from build123d import *

# Parameters (mm, degrees)
SKETCH1_W           = 35.999968648
SKETCH1_H           = 39.60056603
BOSS_EXTRUDE1_DEPTH = 33.93
SKETCH2_W           = 28.93
SKETCH2_H           = 5
SKETCH2_H_2         = 4
CUT_EXTRUDE1_DEPTH  = 64.367558518
SKETCH3_W           = 16
SKETCH3_H           = 5
SKETCH3_H_2         = 4
CUT_EXTRUDE2_DEPTH  = 64.367558518
CUT_EXTRUDE3_DEPTH  = 61.369212453
SKETCH5_W           = 30.4
SKETCH5_H           = 7.2
CUT_EXTRUDE4_DEPTH  = 30.93
CUT_EXTRUDE5_DEPTH  = 62.813165851
BOSS_EXTRUDE2_REACH = 65.368
BOSS_EXTRUDE3_DEPTH = 5
BOSS_EXTRUDE4_REACH = 56.06
BOSS_EXTRUDE5_DEPTH = 5
BOSS_EXTRUDE6_DEPTH = 3
SKETCH12_W          = 35.999968648
SKETCH12_H          = 45.60056603
CUT_EXTRUDE6_DEPTH  = 2
SKETCH13_W          = 30.4
SKETCH13_H          = 39.6
SKETCH13_W_2        = 29.9
SKETCH13_H_2        = 39.1
CUT_EXTRUDE7_DEPTH  = 2


with BuildPart() as part:
    # Sketch1 → Boss-Extrude1 (new body)
    with BuildSketch(Plane.XY):
        with Locations((17.999984324, 19.800283015)):
            Rectangle(SKETCH1_W, SKETCH1_H)
    extrude(amount=-BOSS_EXTRUDE1_DEPTH)

    # Sketch2 → Cut-Extrude1 (cut, through all)
    with BuildSketch(Plane(origin=(35.999968648, 0, 0), x_dir=(0, 0, -1), z_dir=(1, 0, 0))):
        with Locations((19.465, 37.10056603)):
            Rectangle(SKETCH2_W, SKETCH2_H)
        with Locations((19.465, 19.800283015)):
            Rectangle(SKETCH2_W, SKETCH2_H_2)
        with Locations((19.465, 2.5)):
            Rectangle(SKETCH2_W, SKETCH2_H)
    extrude(amount=-CUT_EXTRUDE1_DEPTH, mode=Mode.SUBTRACT)

    # Sketch3 → Cut-Extrude2 (cut, through all)
    with BuildSketch(Plane.XY):
        with Locations((17.999984324, 37.10056603)):
            Rectangle(SKETCH3_W, SKETCH3_H)
        with Locations((17.999984324, 19.800283015)):
            Rectangle(SKETCH3_W, SKETCH3_H_2)
        with Locations((17.999984324, 2.5)):
            Rectangle(SKETCH3_W, SKETCH3_H)
    extrude(amount=-CUT_EXTRUDE2_DEPTH, mode=Mode.SUBTRACT)

    # Sketch4 → Cut-Extrude3 (cut, through all)
    with BuildSketch(Plane(origin=(0, 34.60056603, 0), x_dir=(1, 0, 0), z_dir=(0, 1, 0))):
        Polygon((9.999984324, 0), (17.999984324, 5), (25.999984324, 0), align=None)
    extrude(amount=-CUT_EXTRUDE3_DEPTH, mode=Mode.SUBTRACT)

    # Sketch5 → Cut-Extrude4 (cut)
    with BuildSketch(Plane.XY):
        with Locations((17.999984324, 11.4)):
            Rectangle(SKETCH5_W, SKETCH5_H)
        with Locations((17.999984324, 28.20056603)):
            Rectangle(SKETCH5_W, SKETCH5_H)
    extrude(amount=-CUT_EXTRUDE4_DEPTH, mode=Mode.SUBTRACT)

    # Sketch6 → Cut-Extrude5 (cut, through all)
    with BuildSketch(Plane.XY.offset(-30.93)):
        with BuildLine():
            Line((15.109984324, 29.66056603), (20.889984324, 29.66056603))
            ThreePointArc((20.889984324, 29.66056603), (22.469984324, 28.08056603), (20.889984324, 26.50056603))
            Line((20.889984324, 26.50056603), (15.109984324, 26.50056603))
            ThreePointArc((15.109984324, 26.50056603), (13.529984324, 28.08056603), (15.109984324, 29.66056603))
        make_face()
        with BuildLine():
            Line((15.109984324, 12.86), (20.889984324, 12.86))
            ThreePointArc((20.889984324, 12.86), (22.469984324, 11.28), (20.889984324, 9.7))
            Line((20.889984324, 9.7), (15.109984324, 9.7))
            ThreePointArc((15.109984324, 9.7), (13.529984324, 11.28), (15.109984324, 12.86))
        make_face()
    extrude(amount=-CUT_EXTRUDE5_DEPTH, mode=Mode.SUBTRACT)

    # Sketch7 → Boss-Extrude2 (add, up to next)
    with BuildSketch(Plane.XY, mode=Mode.PRIVATE) as boss_extrude2_sk1:
        Polygon((2.799984324, 28.422935376), (2.799984324, 27.45056603), (3.299984324, 27.45056603), (3.299984324, 27.896781183), align=None)
    boss_extrude2_tool1 = extrude(boss_extrude2_sk1.sketch, amount=-BOSS_EXTRUDE2_REACH, mode=Mode.PRIVATE) - part.part
    # Sketch7 → Boss-Extrude2 (add, up to next)
    with BuildSketch(Plane.XY, mode=Mode.PRIVATE) as boss_extrude2_sk2:
        Polygon((2.799984324, 11.622369346), (2.799984324, 10.65), (3.299984324, 10.65), (3.299984324, 11.096215154), align=None)
    boss_extrude2_tool2 = extrude(boss_extrude2_sk2.sketch, amount=-BOSS_EXTRUDE2_REACH, mode=Mode.PRIVATE) - part.part
    boss_extrude2_1 = boss_extrude2_tool1.solids().sort_by_distance((3.019076, 27.821475, 0))[0]
    add(boss_extrude2_1)
    boss_extrude2_2 = boss_extrude2_tool2.solids().sort_by_distance((3.019076, 11.020909, 0))[0]
    add(boss_extrude2_2)
    boss_extrude2 = boss_extrude2_1 + boss_extrude2_2  # Boss-Extrude2 as one shape, for the pattern or mirror that repeats it

    # Mirror1: Boss-Extrude2 across plane
    add(boss_extrude2.mirror(Plane(origin=(17.999984324, 0, 0), x_dir=(0, 0, 1), z_dir=(1, 0, 0))))

    # Sketch8 → Boss-Extrude3 (add)
    with BuildSketch(Plane(origin=(0, 34.60056603, 0), x_dir=(1, 0, 0), z_dir=(0, 1, 0))):
        Polygon((9.999984324, 5), (17.999984324, 10), (25.999984324, 5), (25.999984324, 0), (17.999984324, 5), (9.999984324, 0), align=None)
    extrude(amount=BOSS_EXTRUDE3_DEPTH)

    # Sketch9 → Boss-Extrude4 (add, up to next)
    with BuildSketch(Plane(origin=(0, 17.800283015, 0), x_dir=(1, 0, 0), z_dir=(0, 1, 0)), mode=Mode.PRIVATE) as boss_extrude4_sk1:
        Polygon((9.999984324, 5), (17.999984324, 10), (25.999984324, 5), (25.999984324, 0), (17.999984324, 5), (9.999984324, 0), align=None)
    boss_extrude4_tool1 = extrude(boss_extrude4_sk1.sketch, amount=BOSS_EXTRUDE4_REACH, mode=Mode.PRIVATE) - part.part
    add(boss_extrude4_tool1.solids().sort_by_distance((14.099984, 17.800283, -7.34))[0])

    # Sketch10 → Boss-Extrude5 (add)
    with BuildSketch(Plane.XZ.offset(-5)):
        Polygon((9.999984324, 0), (17.999984324, -5), (25.999984324, 0), (25.999984324, -5), (17.999984324, -10), (9.999984324, -5), align=None)
    extrude(amount=BOSS_EXTRUDE5_DEPTH)

    # Sketch11 → Boss-Extrude6 (add)
    with BuildSketch(Plane(origin=(0, 39.60056603, 0), x_dir=(1, 0, 0), z_dir=(0, 1, 0))):
        Polygon((0, 5), (9.999984324, 5), (17.999984324, 10), (25.999984324, 5), (35.999968648, 5), (35.999968648, 0), (0, 0), align=None)
    boss_extrude6 = extrude(amount=BOSS_EXTRUDE6_DEPTH)

    # Mirror2: Boss-Extrude6 across plane
    add(boss_extrude6.mirror(Plane.ZX.offset(19.800283015)))

    # Sketch12 → Cut-Extrude6 (cut)
    with BuildSketch(Plane.XY):
        with Locations((17.999984324, 19.800283015)):
            Rectangle(SKETCH12_W, SKETCH12_H)
        Polygon((2.799984324, 39.600283015), (33.199984324, 39.600283015), (33.199984324, 28.422935376), (32.699984324, 27.896781183), (32.699984324, 27.45056603), (33.199984324, 27.45056603), (33.199984324, 11.622369346), (32.699984324, 11.096215154), (32.699984324, 10.65), (33.199984324, 10.65), (33.199984324, 0.000283015), (2.799984324, 0.000283015), (2.799984324, 10.65), (3.299984324, 10.65), (3.299984324, 11.096215154), (2.799984324, 11.622369346), (2.799984324, 27.45056603), (3.299984324, 27.45056603), (3.299984324, 27.896781183), (2.799984324, 28.422935376), align=None, mode=Mode.SUBTRACT)
    extrude(amount=-CUT_EXTRUDE6_DEPTH, mode=Mode.SUBTRACT)

    # Sketch13 → Cut-Extrude7 (cut)
    with BuildSketch(Plane.XY):
        with Locations((17.999984324, 19.800283015)):
            Rectangle(SKETCH13_W, SKETCH13_H)
        with Locations((17.999984324, 19.800283015)):
            Rectangle(SKETCH13_W_2, SKETCH13_H_2, mode=Mode.SUBTRACT)
    extrude(amount=-CUT_EXTRUDE7_DEPTH, mode=Mode.SUBTRACT)


solid = part.part
Verification items for the finished model (mm, model axes). A direction names the side the tool comes from. Coordinates: 2 decimals unless noted, no trailing zeros. Order: outer loops, then holes, each group sorted by start corner. A loop starts at its lowest first (then second) coordinate and runs counter-clockwise, first axis right, second up.
Item 1: Section check C-C, the plane y = 6.5. Enter the section's corners in (x, z), then the cut area to 3 significant figures.
Filled in:
outline: (0, -33.93) - (36, -33.93) - (36, -2) - (32.95, -2) - (32.95, 0) - (26, 0) - (18, -5) - (10, 0) - (3.05, 0) - (3.05, -2) - (0, -2) - close
area: 1,170 mm2
Item 2: Material ranges on L1, parallel to Y at x = 7.5, z = -10; L2, parallel to Y at x = 9.5, z = -4; L3, parallel to X at y = 27.5, z = -11, recorded low to high.
Filled in:
L1: y = 5 to 7.8, 15 to 17.8, 21.8 to 24.6, 31.8 to 34.6
L2: y = -3 to 7.8, 15 to 24.6, 31.8 to 42.6
L3: x = 0 to 3.3, 32.7 to 36
Item 3: Access from +Z, -Z, +X, -X, +Y, -Y to the whole of each face (thin tool, end or side, straight path). Record for faces 1 (the face through (5, 39, -5)), 2 (the face through (18, 30, -33.93)), 3 (the face through (22.47, 28.12, -32.41)), 4 (the face through (2.8, 9, -16)), 5 (the face through (31, 39, -5)).
Filled in:
face 1: -Z, -X, +Y
face 2: -Z, +X, -X, +Y, -Y
face 3: +Z, -Z
face 4: +Z
face 5: -Z, +X, +Y
Item 4: Section check A-A, the plane z = -15.5. Give the number of separate pieces and of enclosed holes in the cut face, then the cut area to 3 significant figures.
Filled in:
separate pieces: 2
enclosed holes: 2
area: 485 mm2
Item 5: Section check D-D, the plane y = 35.5. Enter the section's corners in (x, z), then the cut area to 3 significant figures.
Filled in:
outline: (0, -5) - (10, -5) - (18, -10) - (26, -5) - (36, -5) - (36, -2) - (32.95, -2) - (32.95, 0) - (26, 0) - (18, -5) - (10, 0) - (3.05, 0) - (3.05, -2) - (0, -2) - close
area: 168 mm2
Item 6: Section check B-B, the plane x = 7. Enter the section's corners in (y, z), then the cut area to 3 significant figures.
Filled in:
outline: (-3, -5) - (5, -5) - (5, -33.93) - (17.8, -33.93) - (17.8, -5) - (21.8, -5) - (21.8, -33.93) - (34.6, -33.93) - (34.6, -5) - (42.6, -5) - (42.6, -2) - (39.35, -2) - (39.35, 0) - (31.8, 0) - (31.8, -30.93) - (24.6, -30.93) - (24.6, 0) - (15, 0) - (15, -30.93) - (7.8, -30.93) - (7.8, 0) - (0.25, 0) - (0.25, -2) - (-3, -2) - close
area: 510 mm2
Item 7: Release check for a two-part mould opening along Y. For faces 6 (the face through (22.056, 35.646, -2.465)), 7 (the face through (3.05, 20, -1)), 8 (the face through (7, 0.25, -1)) record: +Y half, -Y half, draft (parallel to the pull), parting line (faces both ways), or undercut.
Filled in:
face 6: undercut
face 7: draft
face 8: -Y half
Item 8: Depth check by flat-ended pin: pin 1 (2 mm diameter, centred on y = 33.5, z = -1.5, fed in from +X); pin 2 (1 mm diameter, centred on y = 19.5, z = -1, fed in from +X); pin 3 (6 mm diameter, centred on x = 21, z = -24, fed in from +Y); pin 4 (2 mm diameter, centred on x = 29.5, z = -27.5, fed in from -Y). Enter the tip coordinate at first touch or a pass-through.
Filled in:
pin 1: stops at x = 36
pin 2: stops at x = 32.95
pin 3: stops at y = 34.6
pin 4: stops at y = 5
